Part model, mm, in its own coordinate system. Face numbers are marked on the shaded views. A direction names the side the tool comes from. Give positions to 0.01 mm unless a question says otherwise; leave off trailing zeros. Write each loop counter-clockwise with the first axis right and the second up, starting at its lowest first coordinate (ties: lowest second). Pieces come first, ordered by that corner, then holes. Notation, with made-up numbers: M 32,42.5 L 70,42.5 A27 ccw 70,73.5 Z; hole C -12.5,21.25 d9. An arc over 180 degrees is marked long. Answer as CSV lines item,"result". Start each with the question number.
1) Slice it at A-A, the plane y = 9.5. Give the cut face in (x, z) (3 decimals), plus the area to 3 significant figures.
2) Tool access for the marked faces 1 and 2: list every direction of +Z, -Z, +X, -X, +Y, -Y with a clear straight run to the whole face (end or side of a thin tool).
3) Slice it at B-B, the plane z = 39.5. Give the cut face in (x, y), plus the area to 3 significant figures.
4) Slice it at C-C, the plane x = 29.5. Give the cut face in (y, z).
5) Slice it at D-D, the plane y = 24. Give the cut face in (x, z) (3 decimals).
6) Pin check, flat tips, straight feed: pin 1 Ø1 at (x, y) = (45, 22.5) entering from -Z; pin 2 Ø12 at (x, y) = (14, 15.5) entering from +Z; pin 3 Ø1.7 at (x, y) = (34, 9) entering from +Z; pin 4 Ø4 at (x, z) = (39.5, 3.5) entering from +Y. Stop position of each tip, or through.
7) Wall check: line 1 along Z through (x, y) = (39.5, 11); line 2 along Y through (x, z) = (34.5, 140); line 3 along Z through (x, y) = (67, 5). Give the ranges that are in metal, low to high. Write a range as from..to.
```python
from build123d import *
from OCP.BRepFilletAPI import BRepFilletAPI_MakeChamfer

# Parameters (mm, degrees)
SKETCH1_W               = 82.55
SKETCH1_H               = 164.338
SKETCH1_R               = 5.08
SKETCH1_R_2             = 1.27
BASE_EXTRUDE_DEPTH      = 2.54
SKETCH6_R               = 2.413
MIDDLE_BAR_HOLDER_DEPTH = 12.7
SKETCH7_R               = 2.55
BOSS_EXTRUDE6_DEPTH     = 27.686
SKETCH7_3_R             = 3.81
SKETCH7_3_R_2           = 2.55
BOSS_EXTRUDE7_DEPTH     = 12.192
CUT_EXTRUDE1_DEPTH      = 10
DRAFT4_ANGLE            = 4
DRAFT5_ANGLE            = 3
CHAMFER1_SIZE           = 0.3
CHAMFER1_SIZE2          = 0.317026351
CHAMFER2_SIZE           = 0.3
CHAMFER2_SIZE2          = 0.317026351
CHAMFER3_SIZE           = 0.3
CHAMFER3_SIZE2          = 0.317026351


with BuildPart() as part:
    # Sketch1 → base extrude (new body)
    with BuildSketch(Plane(origin=(0, 0, 0), x_dir=(1, 0, 0), z_dir=(0, 1, 0))):
        with Locations((41.275, -82.169)):
            Rectangle(SKETCH1_W, SKETCH1_H)
        with Locations(Location((41.275, -58.1000108, 0), (0, 0, 270))):
            Circle(SKETCH1_R, mode=Mode.SUBTRACT)
        with Locations(Location((57.023, -42.3520108, 0), (0, 0, 270))):
            Circle(SKETCH1_R_2, mode=Mode.SUBTRACT)
        with Locations(Location((57.023, -73.8480108, 0), (0, 0, 270))):
            Circle(SKETCH1_R_2, mode=Mode.SUBTRACT)
        with Locations(Location((25.527, -73.8480108, 0), (0, 0, 270))):
            Circle(SKETCH1_R_2, mode=Mode.SUBTRACT)
        with Locations(Location((25.527, -42.3520108, 0), (0, 0, 270))):
            Circle(SKETCH1_R_2, mode=Mode.SUBTRACT)
    extrude(amount=BASE_EXTRUDE_DEPTH)

    # Sketch6 → middle bar holder (add)
    with BuildSketch(Plane(origin=(0, 2.54, 0), x_dir=(1, 0, 0), z_dir=(0, 1, 0))):
        Polygon((33.528, -9.906), (33.528, -4.826), (35.052, -4.826), (37.338, -7.366), (37.338, -9.906), (37.338, -12.446), (35.052, -14.986), (33.528, -14.986), align=None)
        with Locations(Location((41.275, -9.906, 0), (0, 0, 270))):
            Circle(SKETCH6_R)
        Polygon((41.275, -2.159), (46.355, -2.159), (46.355, -3.683), (43.815, -5.969), (41.275, -5.969), (38.735, -5.969), (36.195, -3.683), (36.195, -2.159), align=None)
        Polygon((47.498, -14.986), (45.212, -12.446), (45.212, -9.906), (45.212, -7.366), (47.498, -4.826), (49.022, -4.826), (49.022, -9.906), (49.022, -14.986), align=None)
        Polygon((41.275, -17.653), (36.195, -17.653), (36.195, -16.129), (38.735, -13.843), (41.275, -13.843), (43.815, -13.843), (46.355, -16.129), (46.355, -17.653), align=None)
    extrude(amount=MIDDLE_BAR_HOLDER_DEPTH)

    # Sketch7 → Boss-Extrude6 (add)
    with BuildSketch(Plane(origin=(0, 2.54, 0), x_dir=(1, 0, 0), z_dir=(0, 1, 0))):
        with Locations(Location((17.399, -102.529, 0), (0, 0, 270))):
            Circle(SKETCH7_R)
        with Locations(Location((41.275, -143.692, 0), (0, 0, 270))):
            Circle(SKETCH7_R)
        with Locations(Location((65.151, -102.529, 0), (0, 0, 270))):
            Circle(SKETCH7_R)
    extrude(amount=BOSS_EXTRUDE6_DEPTH)

    # Sketch7<3> → Boss-Extrude7 (add)
    # profile 1 of 3: a face of its own
    with BuildSketch(Plane(origin=(0, 2.54, 0), x_dir=(1, 0, 0), z_dir=(0, 1, 0))):
        with Locations(Location((41.275, -143.692, 0), (0, 0, 90))):
            Circle(SKETCH7_3_R)
        with Locations(Location((41.275, -143.692, 0), (0, 0, 270))):
            Circle(SKETCH7_3_R_2, mode=Mode.SUBTRACT)
    # profile 2 of 3: a face of its own
    with BuildSketch(Plane(origin=(0, 2.54, 0), x_dir=(1, 0, 0), z_dir=(0, 1, 0))):
        with Locations(Location((65.151, -102.529, 0), (0, 0, 90))):
            Circle(SKETCH7_3_R)
        with Locations(Location((65.151, -102.529, 0), (0, 0, 270))):
            Circle(SKETCH7_3_R_2, mode=Mode.SUBTRACT)
    # profile 3 of 3: a face of its own
    with BuildSketch(Plane(origin=(0, 2.54, 0), x_dir=(1, 0, 0), z_dir=(0, 1, 0))):
        with Locations(Location((17.399, -102.529, 0), (0, 0, 90))):
            Circle(SKETCH7_3_R)
        with Locations(Location((17.399, -102.529, 0), (0, 0, 270))):
            Circle(SKETCH7_3_R_2, mode=Mode.SUBTRACT)
    extrude(amount=BOSS_EXTRUDE7_DEPTH)

    # Sketch8 → Cut-Extrude1 (cut)
    with BuildSketch(Plane(origin=(0, 2.54, 0), x_dir=(1, 0, 0), z_dir=(0, 1, 0))):
        Polygon((0, -164.338), (37.384522851, -164.338), (0, -106.566701997), align=None)
        Polygon((82.55, -106.566701997), (45.165477149, -164.338), (82.55, -164.338), align=None)
        Polygon((58.654991564, 0), (82.55, -98.406378462), (82.55, 0), align=None)
        Polygon((0, 0), (0, -98.406378462), (23.895008436, 0), align=None)
    extrude(amount=-CUT_EXTRUDE1_DEPTH, mode=Mode.SUBTRACT)

    # Draft4
    draft4_faces = [part.faces().sort_by_distance(p)[0] for p in [
        (41.275, 8.636, 147.502),
        (17.399, 8.636, 106.339),
        (65.151, 8.636, 106.339),
    ]]
    draft(draft4_faces, Plane.ZX.offset(2.54), DRAFT4_ANGLE)

    # Draft5
    draft5_faces = [part.faces().sort_by_distance(p)[0] for p in [
        (41.275, 8.636, 147.075726154),
        (65.151, 8.636, 105.912726154),
        (17.399, 8.636, 105.912726154),
    ]]
    draft(draft5_faces, Plane.ZX.offset(2.54), DRAFT5_ANGLE)

    # Chamfer1: one chamfer whose edges measure the first distance from different faces: ONE call of the kernel's chamfer builder (chamfer() names one face for all edges)
    chamfer1_edges_1 = [part.edges().sort_by_distance(p)[0] for p in [
        (65.151, 14.732, 99.979),
    ]]
    chamfer1_edges_2 = [part.edges().sort_by_distance(p)[0] for p in [
        (65.151, 2.54, 106.339),
    ]]
    chamfer1_side_2 = [part.faces().sort_by_distance(p)[0] for p in [
        (65.151, 8.636, 106.019522177),
    ]]
    chamfer1_edges_3 = [part.edges().sort_by_distance(p)[0] for p in [
        (65.151, 14.732, 105.700044355),
    ]]
    chamfer1_side_3 = [part.faces().sort_by_distance(p)[0] for p in [
        (65.151, 14.732, 105.610353676),
    ]]
    chamfer1 = BRepFilletAPI_MakeChamfer(part.part.solid().wrapped)
    for e in chamfer1_edges_1:
        chamfer1.Add(CHAMFER1_SIZE, e.wrapped)
    for e in chamfer1_edges_2:
        chamfer1.Add(CHAMFER1_SIZE, CHAMFER1_SIZE2, e.wrapped, chamfer1_side_2[0].wrapped)  # the first distance lies on this face
    for e in chamfer1_edges_3:
        chamfer1.Add(CHAMFER1_SIZE, CHAMFER1_SIZE2, e.wrapped, chamfer1_side_3[0].wrapped)  # the first distance lies on this face
    add(Compound.cast(chamfer1.Shape()), mode=Mode.REPLACE)

    # Chamfer2: one chamfer whose edges measure the first distance from different faces: ONE call of the kernel's chamfer builder (chamfer() names one face for all edges)
    chamfer2_edges_1 = [part.edges().sort_by_distance(p)[0] for p in [
        (17.399, 14.732, 99.979),
    ]]
    chamfer2_edges_2 = [part.edges().sort_by_distance(p)[0] for p in [
        (17.399, 2.54, 106.339),
    ]]
    chamfer2_side_2 = [part.faces().sort_by_distance(p)[0] for p in [
        (41.253202906, 2.54, 80.858952194),
    ]]
    chamfer2_edges_3 = [part.edges().sort_by_distance(p)[0] for p in [
        (17.399, 14.732, 105.700044355),
    ]]
    chamfer2_side_3 = [part.faces().sort_by_distance(p)[0] for p in [
        (17.399, 8.636, 106.019522177),
    ]]
    chamfer2 = BRepFilletAPI_MakeChamfer(part.part.solid().wrapped)
    for e in chamfer2_edges_1:
        chamfer2.Add(CHAMFER2_SIZE, e.wrapped)
    for e in chamfer2_edges_2:
        chamfer2.Add(CHAMFER2_SIZE, CHAMFER2_SIZE2, e.wrapped, chamfer2_side_2[0].wrapped)  # the first distance lies on this face
    for e in chamfer2_edges_3:
        chamfer2.Add(CHAMFER2_SIZE, CHAMFER2_SIZE2, e.wrapped, chamfer2_side_3[0].wrapped)  # the first distance lies on this face
    add(Compound.cast(chamfer2.Shape()), mode=Mode.REPLACE)

    # Chamfer3: one chamfer whose edges measure the first distance from different faces: ONE call of the kernel's chamfer builder (chamfer() names one face for all edges)
    chamfer3_edges_1 = [part.edges().sort_by_distance(p)[0] for p in [
        (41.275, 14.732, 141.142),
    ]]
    chamfer3_edges_2 = [part.edges().sort_by_distance(p)[0] for p in [
        (41.275, 2.54, 147.502),
    ]]
    chamfer3_side_2 = [part.faces().sort_by_distance(p)[0] for p in [
        (41.27378406, 2.54, 80.840255506),
    ]]
    chamfer3_edges_3 = [part.edges().sort_by_distance(p)[0] for p in [
        (41.275, 14.732, 146.863044355),
    ]]
    chamfer3_side_3 = [part.faces().sort_by_distance(p)[0] for p in [
        (41.275, 8.636, 147.182522177),
    ]]
    chamfer3 = BRepFilletAPI_MakeChamfer(part.part.solid().wrapped)
    for e in chamfer3_edges_1:
        chamfer3.Add(CHAMFER3_SIZE, e.wrapped)
    for e in chamfer3_edges_2:
        chamfer3.Add(CHAMFER3_SIZE, CHAMFER3_SIZE2, e.wrapped, chamfer3_side_2[0].wrapped)  # the first distance lies on this face
    for e in chamfer3_edges_3:
        chamfer3.Add(CHAMFER3_SIZE, CHAMFER3_SIZE2, e.wrapped, chamfer3_side_3[0].wrapped)  # the first distance lies on this face
    add(Compound.cast(chamfer3.Shape()), mode=Mode.REPLACE)


solid = part.part
```
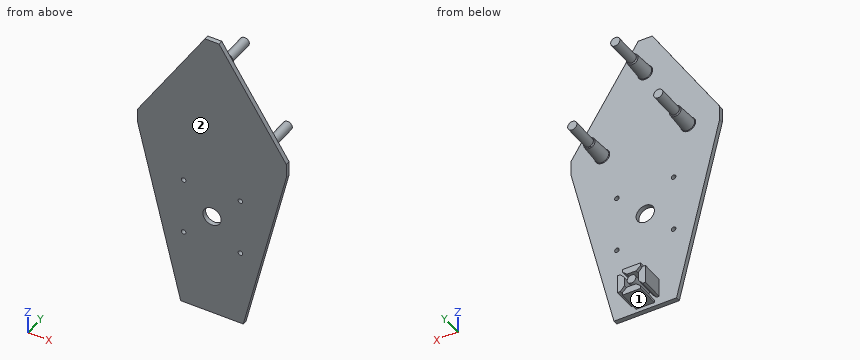
Found:
1,outline,"C 17.399,102.529 d6.89; M 33.528,4.826 L 35.052,4.826 L 37.338,7.366 L 37.338,12.446 L 35.052,14.986 L 33.528,14.986 Z; M 36.195,2.159 L 46.355,2.159 L 46.355,3.683 L 43.815,5.969 L 38.735,5.969 L 36.195,3.683 Z; M 36.195,16.129 L 38.735,13.843 L 43.815,13.843 L 46.355,16.129 L 46.355,17.653 L 36.195,17.653 Z; C 41.275,143.692 d6.89; C 41.275,9.906 d4.826; M 45.212,7.366 L 47.498,4.826 L 49.022,4.826 L 49.022,14.986 L 47.498,14.986 L 45.212,12.446 Z; C 65.151,102.529 d6.89"
1,area,"262 mm²"
2,face 1,"-Z, +X, -X, +Y"
2,face 2,"+Z, -Z, +X, -X, -Y"
3,outline,"M 14.3,0 L 68.25,0 L 68.25,2.54 L 14.3,2.54 Z"
3,area,"137 mm²"
4,outline,"M 0,0 L 2.54,0 L 2.54,152.15 L 0,152.15 Z"
5,outline,"C 17.399,102.529 d5.1; C 41.275,143.692 d5.1; C 65.151,102.529 d5.1"
6,pin 1,"through"
6,pin 2,"z = 105.92"
6,pin 3,"z = 14.99"
6,pin 4,"y = 15.24"
7,line 1,"2.16..5.97, 8.27..11.54, 13.84..17.65, 140.83..146.55"
7,line 2,"0..2.54"
7,line 3,"99.35..105.71"
